from build123d import *

# Parameters (mm, degrees)
SKETCH_R        = 5
PAD_DEPTH       = 4
CHAMFER_SIZE    = 1
CHAMFER001_SIZE = 1
CHAMFER002_SIZE = 1


with BuildPart() as part:
    # Sketch → Pad (new body)
    with BuildSketch(Plane.XY):
        with BuildLine():
            ThreePointArc((-36.75, 15), (-51.75, 0), (-36.75, -15))
            Line((-36.75, -15), (36.75, -15))
            ThreePointArc((36.75, -15), (51.75, 0), (36.75, 15))
            Line((-36.75, 15), (36.75, 15))
        make_face()
        with Locations((-36.75, 0)):
            Circle(SKETCH_R, mode=Mode.SUBTRACT)
        with Locations((36.75, 0)):
            Circle(SKETCH_R, mode=Mode.SUBTRACT)
        with BuildLine():
            ThreePointArc((-11.85289, 9), (-20.85289, 0), (-11.85289, -9))
            Line((-11.85289, -9), (11.85289, -9))
            ThreePointArc((11.85289, -9), (20.85289, 0), (11.85289, 9))
            Line((-11.85289, 9), (11.85289, 9))
        make_face(mode=Mode.SUBTRACT)
    extrude(amount=PAD_DEPTH)

    # Chamfer
    chamfer_edges = [part.edges().sort_by_distance(p)[0] for p in [
        (-41.75, 0, 4),
        (31.75, 0, 4),
    ]]
    chamfer(chamfer_edges, length=CHAMFER_SIZE)

    # Chamfer001
    chamfer001_edges = [part.edges().sort_by_distance(p)[0] for p in [
        (0, 15, 4),
        (51.75, 0, 4),
        (0, -15, 4),
        (-51.75, 0, 4),
    ]]
    chamfer(chamfer001_edges, length=CHAMFER001_SIZE)

    # Chamfer002
    chamfer002_edges = [part.edges().sort_by_distance(p)[0] for p in [
        (20.85289, 0, 4),
        (0, -9, 4),
        (-20.85289, 0, 4),
        (0, 9, 4),
    ]]
    chamfer(chamfer002_edges, length=CHAMFER002_SIZE)


solid = part.part
Design review of the part built by this model. Coordinates are the model's own, in mm. A direction names the side the tool comes from. Coordinates: 2 decimals unless noted, no trailing zeros. Loops run counter-clockwise (first coordinate to the right, second up) from the corner with the lowest first, then second, coordinate; pieces in that order, holes last. Notation, with made-up numbers: M 21,30 L 53,30 A19 cw 53,41 Z; hole C -17,54 d9. An arc over 180 degrees is marked long. Answer as CSV lines item,"result".
Item 1: The part is to be moulded in two halves that separate along X. For faces 1 (the face through (50.92, 0.312, 3.826)), 2 (the face through (-50.92, -0.312, 3.826)), 3 (the face through (0, -9, 1)), 4 (the face through (-1, -15, 1)), say which applies: pulls with the +X half, pulls with the -X half, needs draft (parallel to the pull), parting line crosses it, or undercut.
Answer list:
face 1,"pulls with the +X half"
face 2,"pulls with the -X half"
face 3,"undercut"
face 4,"needs draft"
Item 2: Machinability: for faces 5 (the face through (-21.01, 0.2, 3.16)), 6 (the face through (0, 9, 1)), 7 (the face through (-51.746, 0.33, 1.479)), which of the approach directions +Z, -Z, +X, -X, +Y, -Y give a long, thin tool a straight path to every point of the face, cutting with its end or side? Answer none if there is none.
Answer list:
face 5,"+Z"
face 6,"+Z, -Z"
face 7,"+Z, -Z, -X"
Item 3: For P1, Ø2, axis at y = -11, z = 1, coming from the +X side; P2, Ø8, axis at x = -36.75, y = 0, coming from the +Z side, all flat-tipped, find the tip position at first contact; note any pin that passes through.
Answer list:
P1,"x = 47.93"
P2,"through"
Item 4: For probe 1 along Y at (x, z) = (36.75, 2.35); probe 2 along Y at (x, z) = (0.5, 2.8); probe 3 along X at (y, z) = (2, 1.45), list the stretches that pass through material, from the lowest coordinate up.
Answer list:
probe 1,"-15 to -5, 5 to 15"
probe 2,"-15 to -9, 9 to 15"
probe 3,"-51.62 to -41.33, -32.17 to -20.63, 20.63 to 32.17, 41.33 to 51.62"
Item 5: Add section A-A on x = 4.5. State the section outline as (y, z) points, plus the area to 3 significant figures.
Answer list:
outline,"M -15,0 L -9,0 L -9,3 L -10,4 L -14,4 L -15,3 Z; M 9,0 L 15,0 L 15,3 L 14,4 L 10,4 L 9,3 Z"
area,"46.0 mm²"
Item 6: Add section B-B on z = 1.75. State the section outline as (x, y) points.
Answer list:
outline,"M -36.75,-15 L 36.75,-15 A15 ccw 36.75,15 L -36.75,15 A15 ccw Z; hole C -36.75,0 d10; hole M -11.85,-9 L 11.85,-9 A9 ccw 11.85,9 L -11.85,9 A9 ccw Z; hole C 36.75,0 d10"
